Read the model definition and answer for the solid it produces. Units are mm, in the model's axes. Face numbers are marked on the shaded views. Give positions to 0.01 mm unless a question says otherwise; leave off trailing zeros. Loops run counter-clockwise (first coordinate to the right, second up) from the corner with the lowest first, then second, coordinate; pieces in that order, holes last. Notation, with made-up numbers: (68, 74.25) - (98, 74.25) arc R18 ccw to (98, 86.25) - close; hole circle Ø5 at (81, 88). An arc over 180 degrees is marked (long way). Put each result on its own line as item: value. Start each with the question number.
1. A cutting plane is placed at A-A, the plane z = -28.25. Determine the outline of the cut face in (x, y).
2. Consider L1, parallel to X at y = 2.25, z = -52.75; L2, parallel to X at y = 2.85, z = -7.75; L3, parallel to X at y = 4, z = -38.5. Determine where each line is inside the solid, lowest interval first. Write a range as from..to.
3. For a pull along X with two mould halves and no side action, classify the marked faces 1 and 2 as released by +X, released by -X, zero draft, split by the parting line, or undercut.
4. Given pin 1 Ø1.5 at (x, z) = (-70.3, -28.25) entering from +Y; pin 2 Ø1 at (y, z) = (0, -40.5) entering from -X; pin 3 Ø2 at (x, y) = (-56, 3) entering from +Z; pin 4 Ø1.5 at (y, z) = (0.5, -40) entering from +X, each flat-ended and moving along its own axis, determine where each tip first touches the part or whether it passes through.
5. A cutting plane is placed at C-C, the plane x = -10.5. Determine the outline of the cut face in (y, z).
6. A cutting plane is placed at B-B, the plane y = -1. Count the separate pieces of the cut face and the enclosed holes in it, plus the area to 3 significant figures.
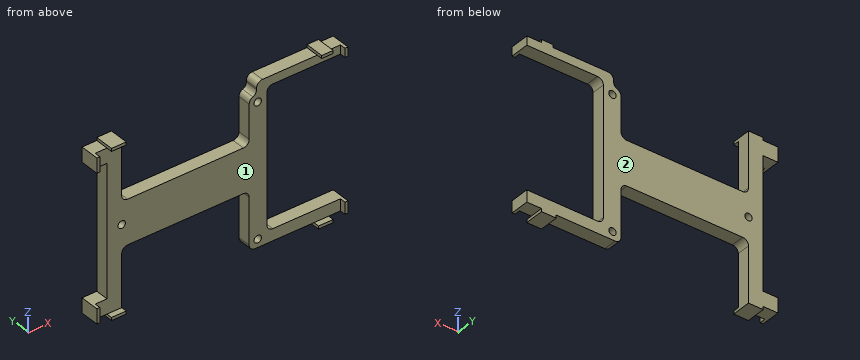
Autodesk Inventor part; units mm, degrees
ref_plane "YZ Plane" through (0, 0, 0) normal (1, 0, 0) x (0, 1, 0)
ref_plane "XZ Plane" through (0, 0, 0) normal (0, 1, 0) x (-1, 0, 0)
ref_plane "XY Plane" through (0, 0, 0) normal (0, 0, 1) x (1, 0, 0)
sketch "Sketch9" plane through (0, 0, 0) normal (0, 1, 0) x (-1, 0, 0)
  line L0 (80.3, -1) -> (75.3, -1)
  line L1 (75.3, -1) -> (75.3, 0)
  line L2 (75.3, 0) -> (70.3, 0)
  line L3 (70.3, 0) -> (70.3, -18.75)
  line L4 (68.3, -20.75) -> (29, -20.75)
  line L5 (0, 0) -> (0, -1)
  line L6 (0, -1) -> (-5, -1)
  line L7 (-5, -1) -> (-5, -4)
  line L8 (-5, -4) -> (19, -4)
  line L9 (21, -6) -> (21, -49.5)
  line L10 (19, -51.5) -> (-5, -51.5)
  line L11 (-5, -51.5) -> (-5, -55.5)
  line L12 (-5, -55.5) -> (0, -55.5)
  line L13 (29, -35.75) -> (68.3, -35.75)
  line L14 (70.3, -37.75) -> (70.3, -56.5)
  line L15 (70.3, -56.5) -> (75.3, -56.5)
  line L16 (75.3, -56.5) -> (75.3, -55.5)
  line L17 (75.3, -55.5) -> (80.3, -55.5)
  line L18 (80.3, -55.5) -> (80.3, -50.5)
  line L19 (80.3, -50.5) -> (75.3, -50.5)
  line L20 (75.3, -50.5) -> (75.3, -6)
  line L21 (75.3, -6) -> (80.3, -6)
  line L22 (80.3, -6) -> (80.3, -1)
  line L23 (27, -37.75) -> (27, -53.5)
  line L24 (25, -55.5) -> (5, -55.5)
  line L25 (0, -55.5) -> (0, -56.5)
  line L26 (0, -56.5) -> (5, -56.5)
  line L27 (5, -56.5) -> (5, -55.5)
  line L28 (3.9072, 0) -> (3.9072, -1)
  line L29 (3.9072, -1) -> (25, -1)
  line L30 (27, -3) -> (27, -18.75)
  line L31 (3.9072, 0) -> (0, 0)
  arc A0 (19, -51.5) -> (21, -49.5) centre (19, -49.5) ccw
  arc A1 (21, -6) -> (19, -4) centre (19, -6) ccw
  arc A2 (27, -3) -> (25, -1) centre (25, -3) ccw
  arc A3 (25, -55.5) -> (27, -53.5) centre (25, -53.5) ccw
  arc A4 (70.3, -37.75) -> (68.3, -35.75) centre (68.3, -37.75) ccw
  arc A5 (68.3, -20.75) -> (70.3, -18.75) centre (68.3, -18.75) ccw
  arc A6 (29, -35.75) -> (27, -37.75) centre (29, -37.75) ccw
  arc A7 (27, -18.75) -> (29, -20.75) centre (29, -18.75) ccw
  point P0 (70.3, -20.75)
  point P1 (27, -20.75)
  point P2 (21, -4)
  point P3 (21, -51.5)
  point P4 (27, -35.75)
  point P5 (70.3, -35.75)
  point P6 (27, -55.5)
  point P7 (27, -1)
  dimension "d42" = 85.3
  dimension "d45" = 15
  dimension "d46" = 5
  dimension "d47" = 5
  dimension "d48" = 5
  dimension "d50" = 1
  dimension "d60" = 4
  dimension "d62" = 26
  dimension "d64" = 1
  dimension "d65" = 5
  dimension "d66" = 5
  dimension "d67" = 6
  dimension "d68" = 3
  dimension "d69" = 56.5
  dimension "d70" = 5
  dimension "d90" = 2
  dimension "d91" = 2
  dimension "d92" = 2
extrude "Extrusion9" add sketch "Sketch9" along normal blind 4.5
sketch "Sketch10" plane through (0, 4.5, 0) normal (0, 1, 0) x (1, 0, 0)
  line L0 (-19, 51.5) -> (5, 51.5)
  line L1 (0, 0) -> (0, 1)
  line L2 (0, 55.5) -> (0, 56.5)
  line L3 (5, 55.5) -> (0, 55.5)
  line L4 (5, 51.5) -> (5, 55.5)
  line L5 (-70.3, 37.75) -> (-70.3, 56.5)
  line L6 (-70.3, 56.5) -> (-75.3, 56.5)
  line L7 (-75.3, 56.5) -> (-75.3, 55.5)
  line L8 (-75.3, 55.5) -> (-80.3, 55.5)
  line L9 (-80.3, 55.5) -> (-80.3, 50.5)
  line L10 (-80.3, 50.5) -> (-75.3, 50.5)
  line L11 (-75.3, 50.5) -> (-75.3, 6)
  line L12 (-75.3, 6) -> (-80.3, 6)
  line L13 (-80.3, 6) -> (-80.3, 1)
  line L14 (-80.3, 1) -> (-75.3, 1)
  line L15 (-75.3, 1) -> (-75.3, 0)
  line L16 (-75.3, 0) -> (-70.3, 0)
  line L17 (-70.3, 0) -> (-70.3, 18.75)
  line L18 (-68.3, 20.75) -> (-29, 20.75)
  line L19 (-27, 18.75) -> (-27, 3)
  line L20 (-25, 1) -> (-3.9072, 1)
  line L21 (-3.9072, 1) -> (-3.9072, 0)
  line L22 (-3.9072, 0) -> (0, 0)
  line L23 (0, 0) -> (0, 1)
  line L24 (0, 1) -> (5, 1)
  line L25 (5, 1) -> (5, 4)
  line L26 (5, 4) -> (-19, 4)
  line L27 (-21, 6) -> (-21, 49.5)
  line L28 (-19, 51.5) -> (5, 51.5)
  line L29 (5, 51.5) -> (5, 55.5)
  line L30 (5, 55.5) -> (0, 55.5)
  line L31 (0, 55.5) -> (0, 56.5)
  line L32 (0, 56.5) -> (-5, 56.5)
  line L33 (-5, 56.5) -> (-5, 55.5)
  line L34 (-5, 55.5) -> (-25, 55.5)
  line L35 (-27, 53.5) -> (-27, 37.75)
  line L36 (-29, 35.75) -> (-68.3, 35.75)
  line L37 (-27, 1) -> (-3.9072, 1)
  line L38 (0, 1) -> (-3.9072, 1)
  line L39 (0, 1) -> (5, 1)
  line L40 (4, 1) -> (4, 4)
  line L41 (5, 4) -> (-21, 4)
  line L42 (4, 51.5) -> (4, 55.5)
  line L43 (-5, 55.5) -> (-27, 55.5)
  line L44 (0, 55.5) -> (-5, 55.5)
  line L45 (-75.3, 55.5) -> (-80.3, 55.5)
  line L46 (-75.3, 55.5) -> (-70.3, 55.5)
  line L47 (-80.3, 1) -> (-75.3, 1)
  line L48 (-79.3, 1) -> (-79.3, 6)
  line L49 (-75.3, 1) -> (-70.3, 1)
  line L50 (-70.3, 0) -> (-70.3, 20.75)
  line L51 (-80.3, 50.5) -> (-75.3, 50.5)
  line L52 (-79.3, 50.5) -> (-79.3, 55.5)
  arc A0 (-68.3, 20.75) -> (-70.3, 18.75) centre (-68.3, 18.75) ccw
  arc A1 (-27, 18.75) -> (-29, 20.75) centre (-29, 18.75) ccw
  arc A2 (-27, 3) -> (-25, 1) centre (-25, 3) ccw
  arc A3 (-21, 6) -> (-19, 4) centre (-19, 6) ccw
  arc A4 (-19, 51.5) -> (-21, 49.5) centre (-19, 49.5) ccw
  arc A5 (-25, 55.5) -> (-27, 53.5) centre (-25, 53.5) ccw
  arc A6 (-29, 35.75) -> (-27, 37.75) centre (-29, 37.75) ccw
  arc A7 (-70.3, 37.75) -> (-68.3, 35.75) centre (-68.3, 37.75) ccw
  point P0 (-75.3, 1)
  dimension "d71" = 1
  dimension "d72" = 1
  dimension "d73" = 1
  dimension "d74" = 1
extrude "Extrusion10" add sketch "Sketch10" against normal blind 6.5 contours L42 L3 L4 L0 | L44 L33 L32 L2 | L26 L25 L24 L40 | L1 L22 L21 L38 | L46 L7 L6 L5 | L52 L10 L9 L8 | L17 L16 L15 L49 | L14 L13 L12 L48
sketch "Sketch11" plane through (0, 4.5, 0) normal (0, 1, 0) x (1, 0, 0)
  line L0 (5, 4) -> (-19, 4)
  line L1 (-21, 6) -> (-21, 49.5)
  line L2 (-19, 51.5) -> (5, 51.5)
  line L3 (5, 51.5) -> (5, 55.5)
  line L4 (5, 55.5) -> (0, 55.5)
  line L5 (0, 55.5) -> (0, 56.5)
  line L6 (0, 56.5) -> (-5, 56.5)
  line L7 (-5, 56.5) -> (-5, 55.5)
  line L8 (-5, 55.5) -> (-25, 55.5)
  line L9 (-27, 53.5) -> (-27, 37.75)
  line L10 (-29, 35.75) -> (-68.3, 35.75)
  line L11 (-70.3, 37.75) -> (-70.3, 56.5)
  line L12 (-70.3, 56.5) -> (-75.3, 56.5)
  line L13 (-75.3, 56.5) -> (-75.3, 55.5)
  line L14 (-75.3, 55.5) -> (-80.3, 55.5)
  line L15 (-80.3, 55.5) -> (-80.3, 50.5)
  line L16 (-80.3, 50.5) -> (-75.3, 50.5)
  line L17 (-75.3, 50.5) -> (-75.3, 6)
  line L18 (-75.3, 6) -> (-80.3, 6)
  line L19 (-80.3, 6) -> (-80.3, 1)
  line L20 (-80.3, 1) -> (-75.3, 1)
  line L21 (-75.3, 1) -> (-75.3, 0)
  line L22 (-75.3, 0) -> (-70.3, 0)
  line L23 (-70.3, 0) -> (-70.3, 18.75)
  line L24 (-68.3, 20.75) -> (-29, 20.75)
  line L25 (-27, 18.75) -> (-27, 3)
  line L26 (-25, 1) -> (-3.9072, 1)
  line L27 (-3.9072, 1) -> (-3.9072, 0)
  line L28 (-3.9072, 0) -> (0, 0)
  line L29 (0, 0) -> (0, 1)
  line L30 (0, 1) -> (5, 1)
  line L31 (5, 1) -> (5, 4)
  circle A0 centre (-70.3, 28.25) radius 1.25
  line L32 (-21, 4) -> (-21, 49.5)
  line L33 (-75.3, 50.5) -> (-75.3, 6)
  arc A1 (-21, 6) -> (-19, 4) centre (-19, 6) ccw
  arc A2 (-19, 51.5) -> (-21, 49.5) centre (-19, 49.5) ccw
  arc A3 (-25, 55.5) -> (-27, 53.5) centre (-25, 53.5) ccw
  arc A4 (-29, 35.75) -> (-27, 37.75) centre (-29, 37.75) ccw
  arc A5 (-70.3, 37.75) -> (-68.3, 35.75) centre (-68.3, 37.75) ccw
  arc A6 (-68.3, 20.75) -> (-70.3, 18.75) centre (-68.3, 18.75) ccw
  arc A7 (-27, 18.75) -> (-29, 20.75) centre (-29, 18.75) ccw
  arc A8 (-27, 3) -> (-25, 1) centre (-25, 3) ccw
  circle A9 centre (-24.1, 7.75) radius 1.25
  circle A10 centre (-24.1, 52.75) radius 1.25
  line L34 (4, 4) -> (4, 1)
  line L35 (0, 1) -> (4, 1)
  line L36 (0, 1) -> (-3.9072, 1)
  line L37 (-25, 1) -> (-3.9072, 1)
  arc A11 (-27, 3) -> (-25, 1) centre (-25, 3) ccw
  line L38 (-27, 18.75) -> (-27, 3)
  arc A12 (-27, 18.75) -> (-29, 20.75) centre (-29, 18.75) ccw
  line L39 (-68.3, 20.75) -> (-29, 20.75)
  arc A13 (-68.3, 20.75) -> (-70.3, 18.75) centre (-68.3, 18.75) ccw
  line L40 (-70.3, 1) -> (-70.3, 18.75)
  line L41 (-70.3, 1) -> (-75.3, 1)
  line L42 (-79.3, 1) -> (-75.3, 1)
  line L43 (-79.3, 1) -> (-79.3, 6)
  line L44 (-75.3, 6) -> (-79.3, 6)
  line L45 (-75.3, 50.5) -> (-75.3, 6)
  line L46 (-79.3, 50.5) -> (-75.3, 50.5)
  line L47 (-79.3, 50.5) -> (-79.3, 55.5)
  line L48 (-75.3, 55.5) -> (-79.3, 55.5)
  line L49 (-75.3, 55.5) -> (-70.3, 55.5)
  line L50 (-70.3, 37.75) -> (-70.3, 55.5)
  arc A14 (-70.3, 37.75) -> (-68.3, 35.75) centre (-68.3, 37.75) ccw
  line L51 (-29, 35.75) -> (-68.3, 35.75)
  arc A15 (-29, 35.75) -> (-27, 37.75) centre (-29, 37.75) ccw
  line L52 (-27, 53.5) -> (-27, 37.75)
  arc A16 (-25, 55.5) -> (-27, 53.5) centre (-25, 53.5) ccw
  line L53 (-5, 55.5) -> (-25, 55.5)
  line L54 (-5, 55.5) -> (0, 55.5)
  line L55 (4, 55.5) -> (0, 55.5)
  line L56 (4, 55.5) -> (4, 51.5)
  line L57 (-19, 51.5) -> (4, 51.5)
  arc A17 (-19, 51.5) -> (-21, 49.5) centre (-19, 49.5) ccw
  line L58 (-21, 6) -> (-21, 49.5)
  arc A18 (-21, 6) -> (-19, 4) centre (-19, 6) ccw
  line L59 (4, 4) -> (-19, 4)
  dimension "d76" = 2.5
  dimension "d93" = 2.5
  dimension "d94" = 2.5
  dimension "d96" = 56.2
  dimension "d97" = 56.2
  dimension "d100" = 7.5
  dimension "d101" = 17
  dimension "d102" = 13
extrude "Extrusion11" cut sketch "Sketch11" against normal through all contours A0 | A9 | A10
sketch "Sketch14" plane through (0, 0, 0) normal (0, -1, 0) x (1, 0, 0)
  circle A0 centre (-70.3, -28.25) radius 1.25
  circle A1 centre (-24.1, -52.75) radius 1.25
  circle A2 centre (-24.1, -7.75) radius 1.25
  line L0 (4, -4) -> (4, -1)
  line L1 (0, -1) -> (4, -1)
  line L2 (0, -1) -> (-3.9072, -1)
  line L3 (-25, -1) -> (-3.9072, -1)
  arc A3 (-25, -1) -> (-27, -3) centre (-25, -3) ccw
  line L4 (-27, -18.75) -> (-27, -3)
  arc A4 (-29, -20.75) -> (-27, -18.75) centre (-29, -18.75) ccw
  line L5 (-68.3, -20.75) -> (-29, -20.75)
  arc A5 (-70.3, -18.75) -> (-68.3, -20.75) centre (-68.3, -18.75) ccw
  line L6 (-70.3, -1) -> (-70.3, -18.75)
  line L7 (-70.3, -1) -> (-75.3, -1)
  line L8 (-79.3, -1) -> (-75.3, -1)
  line L9 (-79.3, -1) -> (-79.3, -6)
  line L10 (-75.3, -6) -> (-79.3, -6)
  line L11 (-75.3, -50.5) -> (-75.3, -6)
  line L12 (-79.3, -50.5) -> (-75.3, -50.5)
  line L13 (-79.3, -50.5) -> (-79.3, -55.5)
  line L14 (-75.3, -55.5) -> (-79.3, -55.5)
  line L15 (-75.3, -55.5) -> (-70.3, -55.5)
  line L16 (-70.3, -37.75) -> (-70.3, -55.5)
  arc A6 (-68.3, -35.75) -> (-70.3, -37.75) centre (-68.3, -37.75) ccw
  line L17 (-29, -35.75) -> (-68.3, -35.75)
  arc A7 (-27, -37.75) -> (-29, -35.75) centre (-29, -37.75) ccw
  line L18 (-27, -53.5) -> (-27, -37.75)
  arc A8 (-27, -53.5) -> (-25, -55.5) centre (-25, -53.5) ccw
  line L19 (-5, -55.5) -> (-25, -55.5)
  line L20 (-5, -55.5) -> (0, -55.5)
  line L21 (4, -55.5) -> (0, -55.5)
  line L22 (4, -55.5) -> (4, -51.5)
  line L23 (-19, -51.5) -> (4, -51.5)
  arc A9 (-21, -49.5) -> (-19, -51.5) centre (-19, -49.5) ccw
  line L24 (-21, -6) -> (-21, -49.5)
  arc A10 (-19, -4) -> (-21, -6) centre (-19, -6) ccw
  line L25 (4, -4) -> (-19, -4)
  line L26 (-27, -18.75) -> (-27, -3)
  line L27 (-25, -1) -> (-3.9072, -1)
  line L28 (-27, -5.5) -> (-26.5, -5.5)
  line L29 (-24.5, -3.5) -> (-24.5, -1)
  line L30 (-24.5, -1) -> (-27, -1)
  line L31 (-27, -1) -> (-27, -5.5)
  arc A11 (-26.5, -5.5) -> (-24.5, -3.5) centre (-26.5, -3.5) ccw
  point P0 (0, 0)
  dimension "d103" = 2
  dimension "d104" = 4.5
  dimension "d105" = 2.5
extrude "Extrusion14" cut sketch "Sketch14" against normal through all contours L29 A11 L28 L4 A3 L3
fillet "Fillet1" radius 2 2 edges at (-27, 2.25, -5.5) (-24.5, 2.25, -1)
properties part number "display_holder_3DPrint"
Return value:
1. outline: (-75.3, 0) - (-71.55, 0) - (-71.55, 4.5) - (-75.3, 4.5) - close; (-69.05, 0) - (-21, 0) - (-21, 4.5) - (-69.05, 4.5) - close
2. L1: x = -80.3..-70.3, -27..-25.35, -22.85..5
2. L2: x = -75.3..-70.3, -27..-25.35, -22.85..-21
2. L3: x = -75.3..-70.3, -27..-21
3. face 1: undercut
3. face 2: zero draft
4. pin 1: passes through
4. pin 2: stops at x = -75.3
4. pin 3: stops at z = -20.75
4. pin 4: stops at x = -21
5. outline: (0, -55.5) - (4.5, -55.5) - (4.5, -51.5) - (0, -51.5) - close; (0, -4) - (4.5, -4) - (4.5, -1) - (0, -1) - close
6. separate pieces: 8
6. enclosed holes: 0
6. area: 35.9 mm2
